Build history of the part. All positions in model axes, mm. Face numbers are marked on the shaded views. Coordinates: 2 decimals unless noted, no trailing zeros. Order: outer loops, then holes, each group sorted by start corner. A loop starts at its lowest first (then second) coordinate and runs counter-clockwise, first axis right, second up. Notation, with made-up numbers: (51, 19.25) - (60, 19.25) arc R25 cw to (60, 37.25) - close; hole circle Ø2 at (24.5, -8). An arc over 180 degrees is marked (long way). Return JSON: item names as keys, results as strings.
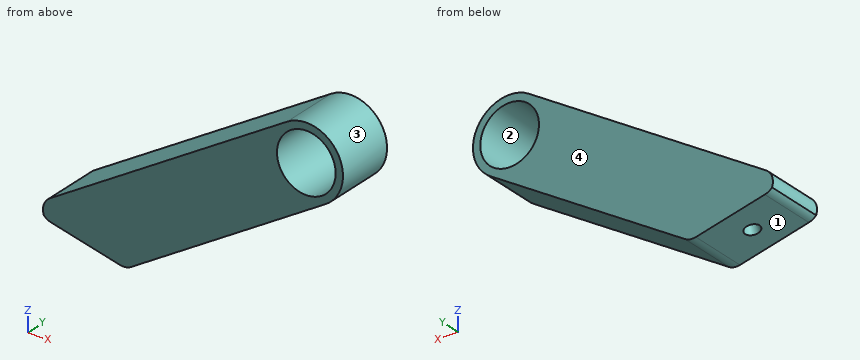
from build123d import *

# Parameters (mm, degrees)
F0_R        = 10
F1_DEPTH    = 20
F2_SIZE     = 20
F4_D        = 5
F4_DEPTH    = 10
F4_TIP      = 1.5021515476
F5_T1_DEPTH = 45
F5_T3_DEPTH = 30.3553390593


# Not quite as in the source:
# - a fillet or chamfer that OpenCascade refuses, or shapes differently, is made with other operations: its cross-section is extruded or revolved along the edge and cut away or added
# - a feature names something its author has since deleted; it is built from what else it names


with BuildPart() as f1:
    # F0 (on Front) → F1 (new body)
    with BuildSketch(Plane.XZ):
        with BuildLine():
            ThreePointArc((11.2991514202, 6.738710196), (15.6399466463, 11.2840038059), (17.2200345341, 17.3672200162))
            ThreePointArc((17.2200345341, 17.3672200162), (10.8032507445, 28.2871321284), (-1.8590823519, 27.9957298365))
            ThreePointArc((-1.8590823519, 27.9957298365), (-5.9084752861, 10.7881031302), (11.2991514202, 6.738710196))
        make_face()
        with Locations((4.7200345341, 17.3672200162)):
            Circle(F0_R, mode=Mode.SUBTRACT)
        with BuildLine():
            ThreePointArc((11.2991514202, 6.738710196), (-5.9084752861, 10.7881031302), (-1.8590823519, 27.9957298365))
            Line((-1.8590823519, 27.9957298365), (-86.8871609141, -24.6372052518))
            Line((-86.8871609141, -24.6372052518), (-73.728927142, -45.8942248924))
            Line((-73.728927142, -45.8942248924), (11.2991514202, 6.738710196))
        make_face()
    extrude(amount=F1_DEPTH)

    # F2
    f2_edges = [f1.edges().sort_by_distance(p)[0] for p in [
        (-73.728927, -10, -45.894225),
    ]]
    chamfer(f2_edges, length=F2_SIZE)

    # F4
    with Locations(Plane(origin=(-10.8625851344, 0, -46.1598350898), x_dir=(0.9734103626, 0, -0.2290682563), z_dir=(-0.2290682563, 0, -0.9734103626))):
        with Locations((-61.2555916321, 10)):
            Hole(F4_D / 2, depth=F4_DEPTH)
            with Locations((0, 0, -(F4_DEPTH + F4_TIP / 2))):  # 118° drill point
                Cone(0, F4_D / 2, F4_TIP, mode=Mode.SUBTRACT)

    # F5: fillet of radius 5 on 3 edges, made by hand

    # F5_s2 → F5_t1 (cut)
    with BuildSketch(Plane.XZ.offset(-12.5)):
        with BuildLine():
            ThreePointArc((-84.2555141597, -28.8886091799), (-84.8711620445, -25.1116211441), (-82.635756986, -22.0055584974))
            Line((-82.635756986, -22.0055584974), (-86.8871609141, -24.6372052518))
            Line((-86.8871609141, -24.6372052518), (-84.2555141597, -28.8886091799))
        make_face()
    extrude(amount=F5_T1_DEPTH, mode=Mode.SUBTRACT)

    # F5_s4 → F5_t3 (cut)
    with BuildSketch(Plane.XZ.offset(-5.1776695297)):
        with BuildLine():
            ThreePointArc((-85.3455779368, -27.1276200138), (-84.0148714695, -28.5542396802), (-82.2395152901, -29.3630250722))
            Line((-82.2395152901, -29.3630250722), (-84.2555141597, -28.8886091799))
            Line((-84.2555141597, -28.8886091799), (-85.3455779368, -27.1276200138))
        make_face()
        with BuildLine():
            ThreePointArc((-58.7393102993, -34.8932219824), (-56.7895862922, -34.9610428559), (-54.9623222634, -34.2775740977))
            Line((-54.9623222634, -34.2775740977), (-56.7233114296, -35.3676378747))
            Line((-56.7233114296, -35.3676378747), (-58.7393102993, -34.8932219824))
        make_face()
    extrude(amount=F5_T3_DEPTH, mode=Mode.SUBTRACT)


solid = f1.part
1. Drop flat-ended pins along their axis: pin 1 (1.5 mm diameter, centred on x = -2, y = -15.5, fed in from -Z); pin 2 (1.5 mm diameter, centred on x = -37, y = -11.5, fed in from +Z); pin 3 (3 mm diameter, centred on y = -13.5, z = 14, fed in from -X). Give the stop position or say it passes through.
Check values:
{"pin 1": "z = -1.96", "pin 2": "z = 6.71", "pin 3": "x = -26.89"}
2. Cut at A-A on z = 9. Give the cut face in (x, y), plus the area to 3 significant figures.
Check values:
{"outline": "(-32.55, -20) - (-0.76, -20) - (-0.76, 0) - (-32.55, 0) - close; (10.2, -20) - (14.01, -20) - (14.01, 0) - (10.2, 0) - close", "area": "712 mm²"}
3. Mould opens along Z. For the marked faces 1, 2, 3 and 4 say: pulls with the +Z half, pulls with the -Z half, needs draft (parallel to the pull), parting line crosses it, or undercut.
Check values:
{"face 1": "pulls with the -Z half", "face 2": "undercut", "face 3": "parting line crosses it", "face 4": "needs draft"}
4. Cut at C-C on y = -15.25. Give the cut face in (x, z).
Check values:
{"outline": "(-84.71, -27.95) arc R5 ccw to (-82.24, -29.36) - (-58.74, -34.89) arc R5 ccw to (-54.96, -34.28) - (11.3, 6.74) arc R12.5 ccw to (-1.86, 28) - (-82.64, -22.01) arc R5 ccw to start; hole circle Ø20 at (4.72, 17.37)"}
5. Cut at D-D on x = -30.5. Give the cut face in (y, z), plus the area to 3 significant figures.
Check values:
{"outline": "(-20, -19.14) - (0, -19.14) - (0, 10.27) - (-20, 10.27) - close", "area": "588 mm²"}
6. Probe L1, parallel to Z at x = 0.5, y = -1.25; L2, parallel to X at y = -11, z = 18; L3, parallel to X at y = -2, z = 19. List the from-to ranges inside material, lowest first.
Check values:
{"L1": "0.05 to 8.3, 26.43 to 29.13", "L2": "-18.01 to -5.26, 14.7 to 17.2", "L3": "-16.39 to -5.15, 14.59 to 17.11"}
7. Cut at B-B on x = 6.5. Give the cut face in (y, z).
Check values:
{"outline": "(-20, 3.77) - (0, 3.77) - (0, 7.53) - (-20, 7.53) - close; (-20, 27.21) - (0, 27.21) - (0, 29.74) - (-20, 29.74) - close"}
